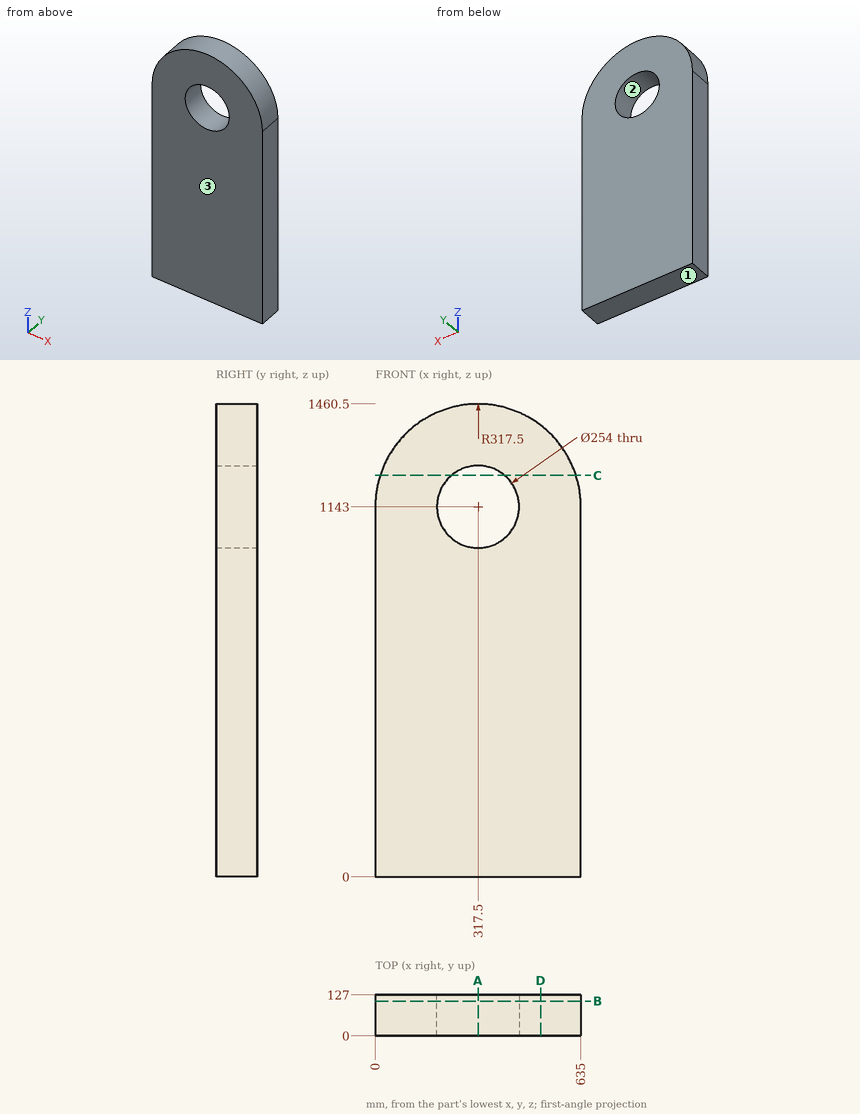
Could you check a few things on this drawing? It's one solid part, dimensions in mm from its lowest x, y, z. Round coordinates to 2 decimals unless told otherwise and drop trailing zeros. Order: outer loops, then holes, each group sorted by start corner. A loop starts at its lowest first (then second) coordinate and runs counter-clockwise, first axis right, second up. Notation, with made-up numbers: M 19.5,2 L 77.5,2 A24 cw 77.5,39 Z; hole C 69.5,36.25 d6. An arc over 180 degrees is marked long. Use a Markdown table: item, result.
1) Imagine slicing it at A-A (x = 317.5). List the corners of the cut face in (y, z) for me.
Geometry says:
| item | result |
|---|---|
| outline | M 0,0 L 127,0 L 127,1016 L 0,1016 Z; M 0,1270 L 127,1270 L 127,1460.5 L 0,1460.5 Z |
2) Imagine slicing it at C-C (z = 1240). List the corners of the cut face in (x, y) for me.
Geometry says:
| item | result |
|---|---|
| outline | M 15.18,0 L 235.52,0 L 235.52,127 L 15.18,127 Z; M 399.48,0 L 619.82,0 L 619.82,127 L 399.48,127 Z |
3) Imagine slicing it at D-D (x = 510.5). List the corners of the cut face in (y, z) for me.
Geometry says:
| item | result |
|---|---|
| outline | M 0,0 L 127,0 L 127,1395.11 L 0,1395.11 Z |
4) Imagine slicing it at B-B (y = 107.5). List the corners of the cut face in (x, z) for me.
Geometry says:
| item | result |
|---|---|
| outline | M 0,0 L 635,0 L 635,1143 A317.5 ccw 0,1143 Z; hole C 317.5,1143 d254 |
5) If we mould it in two halves opening along Z, with no side actions, what happens to the marked faces 1, 2 and 3? For each: +Z half, -Z half, draft (parallel to the pull), parting line (faces both ways), or undercut.
Geometry says:
| item | result |
|---|---|
| face 1 | -Z half |
| face 2 | undercut |
| face 3 | draft |
6) I'm going to push flat-ended pins straight in: P1, Ø2, axis at x = 183.5, y = 90, coming from the +Z side; P2, Ø2, axis at x = 197.5, y = 111, coming from the +Z side; P3, Ø2, axis at y = 105, z = 1245.5, coming from the +X side. Where does each tip first touch, or does it pass through?
Geometry says:
| item | result |
|---|---|
| P1 | stops at z = 1431.3 |
| P2 | stops at z = 1437.36 |
| P3 | stops at x = 618.34 |
7) If I drill on line 1 along Z through (x, y) = (317.5, 53.5); line 2 along X through (y, z) = (112, 1154); line 3 along Z through (x, y) = (259, 81.5), over which ranges is the centre line in solid material (lowest first)?
Geometry says:
| item | result |
|---|---|
| line 1 | z = 0 to 1016, 1270 to 1460.5 |
| line 2 | x = 0.19 to 190.98, 444.02 to 634.81 |
| line 3 | z = 0 to 1030.28, 1255.72 to 1455.06 |
